Input: dimensioned drawing with shaded views. Units: mm. Origin: part minimum x, y, z. Round coordinates to 2 decimals unless told otherwise and drop trailing zeros. Loops run counter-clockwise (first coordinate to the right, second up) from the corner with the lowest first, then second, coordinate; pieces in that order, holes last. Notation, with made-up numbers: (-34.5, 57) - (-4.5, 57) arc R24 cw to (-4.5, 79) - close; hole circle Ø11 at (-20, 0.25). An arc over 180 degrees is marked (long way). Answer as a JSON object with one key per item and string values. Group by question number.
Item 1: Section B-B (x = 2.4). Return the cut outline in (y, z).
Item 2: Section A-A (y = 21.5). Return the cut outline in (x, z), plus the area to 3 significant figures.
Item 3: Line query: line 1 (Z direction, x = 0.2, y = 21.5); line 2 (Y direction, x = 2.1, z = 48.5). Output: solid intervals per line, ascending.
Item 4: Section C-C (z = 45). Return the cut outline in (x, y), plus the area to 3 significant figures.
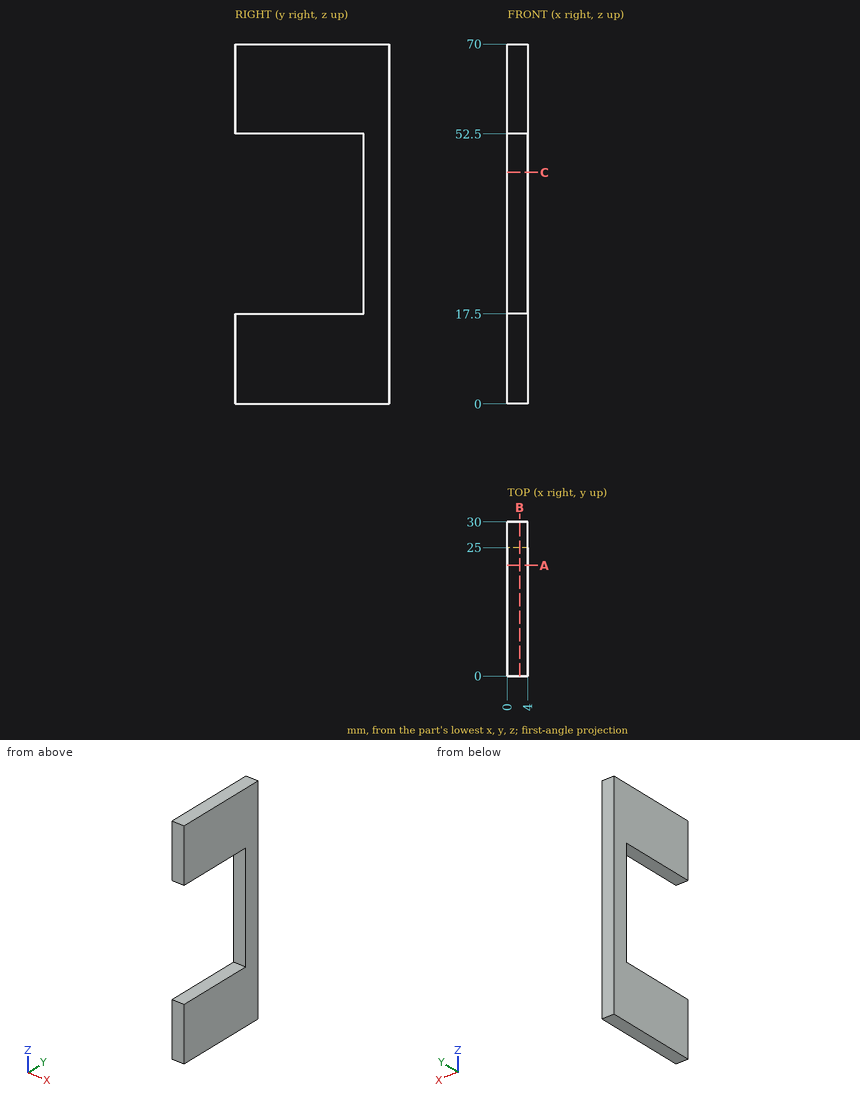
Values:
{
 "1": {"outline": "(0, 0) - (30, 0) - (30, 70) - (0, 70) - (0, 52.5) - (25, 52.5) - (25, 17.5) - (0, 17.5) - close"},
 "2": {"outline": "(0, 0) - (4, 0) - (4, 17.5) - (0, 17.5) - close; (0, 52.5) - (4, 52.5) - (4, 70) - (0, 70) - close", "area": "140 mm^2"},
 "3": {"line 1": "z = 0 to 17.5, 52.5 to 70", "line 2": "y = 25 to 30"},
 "4": {"outline": "(0, 25) - (4, 25) - (4, 30) - (0, 30) - close", "area": "20.0 mm^2"}
}
